```python
from build123d import *

# Parameters (mm, degrees)
F1_DEPTH = 2
F4_DEPTH = 130.110583
F5_W     = 3
F5_H     = 2
F6_DEPTH = 1.5


with BuildPart() as f1:
    # F0 (on Top) → F1 (new body)
    with BuildSketch(Plane.XY):
        Polygon((-70.511212, -40.909583), (0, 0), (0, 70), (-70.511212, -0.909583), align=None)
    extrude(amount=F1_DEPTH)

    # F3 (on offset) → F4 (cut, through all)
    with BuildSketch(Plane.XZ.offset(-89.2)):
        Polygon((-70.511212, 0), (0, 0), (-70.511212, 0.75), align=None)
        Polygon((-70.511212, 1.25), (0, 2), (-70.511212, 2), align=None)
    extrude(amount=F4_DEPTH, mode=Mode.SUBTRACT)

    # F5 (on face) → F6 (join)
    with BuildSketch(Plane.YZ):
        with Locations((58.5, 1)):
            Rectangle(F5_W, F5_H)
        with Locations((11.5, 1)):
            Rectangle(F5_W, F5_H)
    extrude(amount=F6_DEPTH)


solid = f1.part
```
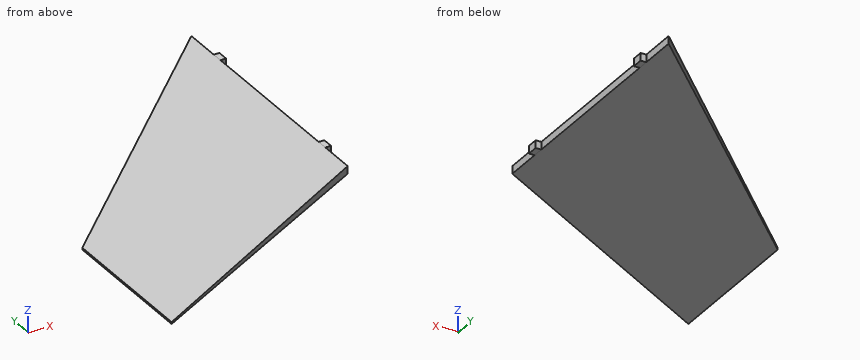
Geometry check sheet. Reference: the model listing, model coordinates, mm. Coordinates: 2 decimals unless noted, no trailing zeros. Write each loop counter-clockwise with the first axis right and the second up, starting at its lowest first coordinate (ties: lowest second). Pieces come first, ordered by that corner, then holes. Notation, with made-up numbers: M 89,10.25 L 103,10.25 A18 ccw 103,41.25 Z; hole C 19,79.5 d4. An arc over 180 degrees is marked long. One line per item, written item: value. Start each with the question number.
(1) Scan lines: line 1 along Y through (x, z) = (-3, 1.15); line 2 along Y through (x, z) = (-19, 0.6); line 3 along Z through (x, y) = (-23.5, 10.5). Record each from-to range of solid material in increasing order. Write a range as [from, to].
(2) Sectioned sample at C-C, the plane y = 39.5. Enter the section's corners in (x, z).
(3) Depth check by flat-ended pin: pin 1 (1.2 mm diameter, centred on x = 1, z = 1, fed in from +Y); pin 2 (6 mm diameter, centred on x = -33.5, y = 36.5, fed in from -Z); pin 3 (1.2 mm diameter, centred on x = 0.5, z = 1, fed in from -Y). Enter the tip coordinate at first touch or a pass-through.
(4) Sectioned sample at A-A, the plane z = 1.6. Enter the section's corners in (x, y), and give its area (3 significant figures).
(5) Sectioned sample at B-B, the plane x = -14. Enter the section's corners in (y, z), and give its area (3 significant figures).
Filled sheet:
1. line 1: [-1.74, 66.98]
1. line 2: [-11.02, 50.89]
1. line 3: [0.25, 1.75]
2. outline: M -30.33,0.32 L 0,0 L 0,2 L -30.33,1.68 Z
3. pin 1: y = 60
3. pin 2: z = 0.32
3. pin 3: y = -0.06
4. outline: M -37.61,-21.82 L 0,0 L 0,10 L 1.5,10 L 1.5,13 L 0,13 L 0,57 L 1.5,57 L 1.5,60 L 0,60 L 0,70 L -37.61,32.18 Z
4. area: 2,340 mm²
5. outline: M -8.12,0.15 L 55.92,0.15 L 55.92,1.85 L -8.12,1.85 Z
5. area: 109 mm²
